The model under review builds one solid part; all positions refer to its coordinate system, in mm. A direction names the side the tool comes from. Give positions to 0.01 mm unless a question says otherwise; leave off trailing zeros. Order: outer loops, then holes, each group sorted by start corner. A loop starts at its lowest first (then second) coordinate and runs counter-clockwise, first axis right, second up.
```python
from build123d import *

# Parameters (mm, degrees)
F0_R     = 11.049
F1_DEPTH = 6.35


with BuildPart() as f1:
    # F0 (on Top) → F1 (new body)
    with BuildSketch(Plane.XY):
        with BuildLine():
            ThreePointArc((-2.36e-08, -13.97), (9.8782817248, -9.8782817415), (13.97, 0))
            ThreePointArc((13.97, 0), (13.8409108955, 1.8947521167), (13.4560292651, 3.754487504))
            ThreePointArc((13.4560292651, 3.754487504), (12.8788953824, 5.4124812914), (12.0983749493, 6.9849998988))
            ThreePointArc((12.0983749493, 6.9849998988), (1.7521013954, 13.8596912195), (-9.9794961892, 9.7760194256))
            ThreePointArc((-9.9794961892, 9.7760194256), (-11.1267940276, 8.4472098748), (-12.0983748995, 6.9849999851))
            ThreePointArc((-12.0983748995, 6.9849999851), (-12.8788953564, -5.4124813532), (-3.4765330758, -13.5305069296))
            ThreePointArc((-3.4765330758, -13.5305069296), (-1.7521013491, -13.8596912254), (-2.36e-08, -13.97))
        make_face()
        Circle(F0_R, mode=Mode.SUBTRACT)
        with BuildLine():
            ThreePointArc((13.4560292651, 3.754487504), (13.8409108955, 1.8947521167), (13.97, 0))
            ThreePointArc((13.97, 0), (9.8782817248, -9.8782817415), (-2.36e-08, -13.97))
            ThreePointArc((-2.36e-08, -13.97), (8.2549999898, -16.1819205776), (14.2980794165, -22.225))
            ThreePointArc((14.2980794165, -22.225), (14.2980794165, -8.255), (26.3964543074, -1.27))
            ThreePointArc((26.3964543074, -1.27), (19.7017499565, 0.1482461704), (14.1572259578, 4.1593236033))
            Line((14.1572259578, 4.1593236033), (13.4560292651, 3.754487504))
        make_face()
        with BuildLine():
            ThreePointArc((12.0983749493, 6.9849998988), (12.8788953824, 5.4124812914), (13.4560292651, 3.754487504))
            Line((13.4560292651, 3.754487504), (14.1572259578, 4.1593236033))
            ThreePointArc((14.1572259578, 4.1593236033), (13.0527933882, 5.5175099241), (12.0983749493, 6.9849998988))
        make_face()
        with BuildLine():
            ThreePointArc((-3.4765330758, -14.3401791282), (-1.7480928878, -14.0628056217), (-2.36e-08, -13.97))
            ThreePointArc((-2.36e-08, -13.97), (-1.7521013491, -13.8596912254), (-3.4765330758, -13.5305069296))
            Line((-3.4765330758, -13.5305069296), (-3.4765330758, -14.3401791282))
        make_face()
        with BuildLine():
            ThreePointArc((-9.9794961892, 9.7760194256), (1.7521013954, 13.8596912195), (12.0983749493, 6.9849998988))
            ThreePointArc((12.0983749493, 6.9849998988), (9.8864543074, 15.2399999416), (12.0983748909, 23.495))
            ThreePointArc((12.0983748909, 23.495), (0, 16.51), (-12.0983748909, 23.495))
            ThreePointArc((-12.0983748909, 23.495), (-9.9792599278, 16.9880928761), (-10.680692882, 10.1808555249))
            Line((-10.680692882, 10.1808555249), (-9.9794961892, 9.7760194256))
        make_face()
        with BuildLine():
            Line((19.5333762679, 7.2632454321), (14.1572259578, 4.1593236033))
            ThreePointArc((14.1572259578, 4.1593236033), (19.7017499565, 0.1482461704), (26.3964543074, -1.27))
            ThreePointArc((26.3964543074, -1.27), (36.2747360405, -5.3617182668), (40.3664543073, -15.24))
            ThreePointArc((40.3664543073, -15.24), (30.0121563674, -28.7339837933), (14.2980794165, -22.225))
            Line((14.2980794165, -22.225), (18.5129530728, -32.0653753202))
            Line((18.5129530728, -32.0653753202), (14.2964770949, -29.5855224255))
            Line((14.2964770949, -29.5855224255), (13.8160917687, -26.1500289008))
            Line((13.8160917687, -26.1500289008), (7.6188843675, -26.0812350595))
            Line((7.6188843675, -26.0812350595), (7.6586053261, -22.5030220397))
            Line((7.6586053261, -22.5030220397), (1.4429174314, -21.1629279691))
            Line((1.4429174314, -21.1629279691), (3.4801004676, -24.6914324922))
            Line((3.4801004676, -24.6914324922), (6.7429192586, -30.342800414))
            Line((6.7429192586, -30.342800414), (12.3789807439, -33.641130461))
            Line((12.3789807439, -33.641130461), (18.9779134399, -37.6940080274))
            Line((18.9779134399, -37.6940080274), (24.2913333671, -32.5875241804))
            Line((24.2913333671, -32.5875241804), (33.0798736321, -35.4493195164))
            Line((33.0798736321, -35.4493195164), (39.4581922442, -29.4734863592))
            Line((39.4581922442, -29.4734863592), (43.9366570858, -23.6116887214))
            Line((43.9366570858, -23.6116887214), (44.0099485225, -16.3618282657))
            Line((44.0099485225, -16.3618282657), (49.9108565981, -16.6858625943))
            Line((49.9108565981, -16.6858625943), (43.1618704508, -11.0453059989))
            Line((43.1618704508, -11.0453059989), (40.7443994954, -2.1940317001))
            Line((40.7443994954, -2.1940317001), (37.0559956245, 4.1944712032))
            Line((37.0559956245, 4.1944712032), (31.3842575072, 5.5065100534))
            Line((31.3842575072, 5.5065100534), (29.1446442552, 12.5378607885))
            Line((29.1446442552, 12.5378607885), (25.7749684952, 7.8452786686))
            Line((25.7749684952, 7.8452786686), (28.8350082813, 4.0347003266))
            Line((28.8350082813, 4.0347003266), (22.6981406857, 4.0953499054))
            Line((22.6981406857, 4.0953499054), (19.5333762679, 7.2632454321))
        make_face()
        with BuildLine():
            Line((-3.4765330758, -14.3401791282), (-3.4765330758, -13.5305069296))
            ThreePointArc((-3.4765330758, -13.5305069296), (-12.8788953564, -5.4124813532), (-12.0983748995, 6.9849999851))
            ThreePointArc((-12.0983748995, 6.9849999851), (-18.1414543148, 0.9419205792), (-26.3964543073, -1.27))
            ThreePointArc((-26.3964543073, -1.27), (-16.5181725742, -5.3617182668), (-12.4264543073, -15.24))
            ThreePointArc((-12.4264543073, -15.24), (-12.9024705141, -18.8557020601), (-14.2980794165, -22.225))
            ThreePointArc((-14.2980794165, -22.225), (-9.7224900287, -17.1363390465), (-3.4765330758, -14.3401791282))
        make_face()
        with BuildLine():
            ThreePointArc((26.3964543074, -1.27), (14.2980794165, -8.255), (14.2980794165, -22.225))
            ThreePointArc((14.2980794165, -22.225), (30.0121563674, -28.7339837933), (40.3664543073, -15.24))
            ThreePointArc((40.3664543073, -15.24), (36.2747360405, -5.3617182668), (26.3964543074, -1.27))
        make_face()
        with Locations((26.3964543073, -15.24)):
            Circle(F0_R, mode=Mode.SUBTRACT)
        with BuildLine():
            Line((-3.4765330758, -20.5480227857), (-3.4765330758, -14.3401791282))
            ThreePointArc((-3.4765330758, -14.3401791282), (-9.7224900287, -17.1363390465), (-14.2980794165, -22.225))
            ThreePointArc((-14.2980794165, -22.225), (-38.4948291982, -22.225), (-26.3964543073, -1.27))
            Line((-26.3964543073, -1.27), (-37.0259061456, 0))
            Line((-37.0259061456, 0), (-32.7700525522, 2.4116488639))
            Line((-32.7700525522, 2.4116488639), (-29.5546352221, 1.1099279977))
            Line((-29.5546352221, 1.1099279977), (-26.3964543073, 6.442470119))
            Line((-26.3964543073, 6.442470119), (-23.3174914114, 4.6189642499))
            Line((-23.3174914114, 4.6189642499), (-19.0490919554, 9.3318608334))
            Line((-19.0490919554, 9.3318608334), (-23.1234580278, 9.3318608334))
            Line((-23.1234580278, 9.3318608334), (-29.6490956098, 9.3318608334))
            Line((-29.6490956098, 9.3318608334), (-35.3235639632, 6.1000534333))
            Line((-35.3235639632, 6.1000534333), (-42.1329252422, 2.4116488639))
            Line((-42.1329252422, 2.4116488639), (-40.3672904702, -4.7431496975))
            Line((-40.3672904702, -4.7431496975), (-47.2399480641, -10.9233511612))
            Line((-47.2399480641, -10.9233511612), (-45.2538840473, -19.4350536913))
            Line((-45.2538840473, -19.4350536913), (-42.4166508019, -26.2444168329))
            Line((-42.4166508019, -26.2444168329), (-36.1747331917, -29.9328193069))
            Line((-36.1747331917, -29.9328193069), (-39.4058091898, -34.8811384415))
            Line((-39.4058091898, -34.8811384415), (-31.146450813, -31.8566232858))
            Line((-31.146450813, -31.8566232858), (-22.2722869366, -34.1886691749))
            Line((-22.2722869366, -34.1886691749), (-14.8954791948, -34.1886691749))
            Line((-14.8954791948, -34.1886691749), (-10.9233511612, -29.9328193069))
            Line((-10.9233511612, -29.9328193069), (-3.7142161756, -31.5089327035))
            Line((-3.7142161756, -31.5089327035), (-6.0932736208, -26.2444168329))
            Line((-6.0932736208, -26.2444168329), (-10.9233511612, -26.9891998532))
            Line((-10.9233511612, -26.9891998532), (-7.8023932874, -21.7048414052))
            Line((-7.8023932874, -21.7048414052), (-3.4765330758, -20.5480227857))
        make_face()
        with BuildLine():
            ThreePointArc((-12.0983748995, 6.9849999851), (-11.1267940276, 8.4472098748), (-9.9794961892, 9.7760194256))
            Line((-9.9794961892, 9.7760194256), (-10.680692882, 10.1808555249))
            ThreePointArc((-10.680692882, 10.1808555249), (-11.3047004812, 8.5452956412), (-12.0983748995, 6.9849999851))
        make_face()
        with BuildLine():
            ThreePointArc((-12.0983748909, 23.495), (0, 16.51), (12.0983748909, 23.495))
            ThreePointArc((12.0983748909, 23.495), (13.4939837933, 26.8642979399), (13.97, 30.48))
            ThreePointArc((13.97, 30.48), (-3.6157020601, 43.9739837933), (-12.0983748909, 23.495))
        make_face()
        with Locations((0, 30.48)):
            Circle(F0_R, mode=Mode.SUBTRACT)
        with BuildLine():
            ThreePointArc((13.97, 30.48), (13.4939837933, 26.8642979399), (12.0983748909, 23.495))
            Line((12.0983748909, 23.495), (18.5129530728, 32.0653753202))
            Line((18.5129530728, 32.0653753202), (18.4735754573, 27.1738735616))
            Line((18.4735754573, 27.1738735616), (15.7385434534, 25.0401009031))
            Line((15.7385434534, 25.0401009031), (18.7775699398, 19.6387649405))
            Line((18.7775699398, 19.6387649405), (15.6588860852, 17.8840577898))
            Line((15.6588860852, 17.8840577898), (17.606174524, 11.8310671357))
            Line((17.606174524, 11.8310671357), (19.6433575602, 15.3595716588))
            Line((19.6433575602, 15.3595716588), (22.9061763512, 21.0109395806))
            Line((22.9061763512, 21.0109395806), (22.9445832193, 27.5410770276))
            Line((22.9445832193, 27.5410770276), (23.1550118023, 35.2823591635))
            Line((23.1550118023, 35.2823591635), (16.0759571031, 37.3306738779))
            Line((16.0759571031, 37.3306738779), (14.160074432, 46.3726706775))
            Line((14.160074432, 46.3726706775), (5.7956918031, 48.9085400505))
            Line((5.7956918031, 48.9085400505), (-1.5200062839, 49.8561055544))
            Line((-1.5200062839, 49.8561055544), (-7.8352153308, 46.2946475726))
            Line((-7.8352153308, 46.2946475726), (-10.5050474083, 51.5670010358))
            Line((-10.5050474083, 51.5670010358), (-12.0154196378, 42.9019292847))
            Line((-12.0154196378, 42.9019292847), (-18.4721125587, 36.382700875))
            Line((-18.4721125587, 36.382700875), (-22.1605164296, 29.9941979717))
            Line((-22.1605164296, 29.9941979717), (-20.460906346, 24.4263092535))
            Line((-20.460906346, 24.4263092535), (-25.4304280796, 18.971071915))
            Line((-25.4304280796, 18.971071915), (-19.6816948744, 18.3991381643))
            Line((-19.6816948744, 18.3991381643), (-17.9116571201, 22.9544995267))
            Line((-17.9116571201, 22.9544995267), (-14.8957473983, 17.6094914998))
            Line((-14.8957473983, 17.6094914998), (-16.0568431921, 13.2847773536))
            Line((-16.0568431921, 13.2847773536), (-10.680692882, 10.1808555249))
            ThreePointArc((-10.680692882, 10.1808555249), (-9.9792599278, 16.9880928761), (-12.0983748909, 23.495))
            ThreePointArc((-12.0983748909, 23.495), (-3.6157020601, 43.9739837933), (13.97, 30.48))
        make_face()
        with BuildLine():
            ThreePointArc((-26.3964543073, -1.27), (-38.4948291982, -22.225), (-14.2980794165, -22.225))
            ThreePointArc((-14.2980794165, -22.225), (-12.9024705141, -18.8557020601), (-12.4264543073, -15.24))
            ThreePointArc((-12.4264543073, -15.24), (-16.5181725742, -5.3617182668), (-26.3964543073, -1.27))
        make_face()
        with Locations((-26.3964543073, -15.24)):
            Circle(F0_R, mode=Mode.SUBTRACT)
    extrude(amount=F1_DEPTH)


solid = f1.part
```
Item 1: Draft analysis for pull direction Y (two halves, no side actions). For faces 5 (the flat face through (-11.25, 47.3, 3.13)), 6 (the flat face through (36.224, -32.503, 3.131)), 7 (the flat face through (16.376, -27.076, 3.131)), state which applies: released by +Y, released by -Y, zero draft, split by the parting line, or undercut.
Values found:
face 5: released by +Y
face 6: released by -Y
face 7: undercut
Item 2: Take a section at C-C (z = 1.75). Give the number of separate pieces and of enclosed holes in the cut face, and give its area (3 significant figures).
Values found:
separate pieces: 1
enclosed holes: 4
area: 2,840 mm2
Item 3: Take a section at B-B (y = 40). Give the boundary of the cut face in (x, z).
Values found:
outline: (-14.89, 0) - (-5.61, 0) - (-5.61, 6.35) - (-14.89, 6.35) - close; (5.61, 0) - (15.51, 0) - (15.51, 6.35) - (5.61, 6.35) - close
Item 4: Clearance check with flat-ended pins moving along their axes: pin 1 Ø20 at (x, y) = (26.4, -15.24) entering from -Z; pin 2 Ø12 at (x, y) = (-13.5, 11.5) entering from +Z; pin 3 Ø1.9 at (y, z) = (-18, 3.5) entering from +X; pin 4 Ø2 at (y, z) = (8.5, 5) entering from -X. State where each tip first meets the part, or that it passes through.
Values found:
pin 1: passes through
pin 2: stops at z = 6.35
pin 3: stops at x = 44
pin 4: stops at x = -32.87
Item 5: Take a section at A-A (y = -6.5). Give the boundary of the cut face in (x, z), and give its area (3 significant figures).
Values found:
outline: (-42.32, 0) - (-33.16, 0) - (-33.16, 6.35) - (-42.32, 6.35) - close; (-19.64, 0) - (-8.93, 0) - (-8.93, 6.35) - (-19.64, 6.35) - close; (8.93, 0) - (19.64, 0) - (19.64, 6.35) - (8.93, 6.35) - close; (33.16, 0) - (41.92, 0) - (41.92, 6.35) - (33.16, 6.35) - close
area: 250 mm2
Item 6: For line 1 (X direction, y = 29, z = 6.25); line 2 (X direction, y = -27.5, z = 1.75); line 3 (Y direction, x = 0, z = 4.75), list the stretches that pass through material, from the lowest coordinate up.
Values found:
line 1: x = -21.86 to -10.95, 10.95 to 16.22, 18.49 to 22.98
line 2: x = -40.29 to -5.53, 5.1 to 14, 16.56 to 40.97
line 3: y = -13.97 to -11.05, 11.05 to 19.43, 41.53 to 49.66
Item 7: For faces 1 (the flat face through (-19, -34.189, 3)), 2 (the flat face through (-4.63, 48.1, 3.13)), 3 (the flat face through (-31.18, 1.77, 3.13)), 4 (the flat face through (-41.26, -1.12, 3.13)), list the 3-axis set-ups (+Z, -Z, +X, -X, +Y, -Y) from which the entire face can be reached by the end or side of a thin tool; tool diameter is ignored.
Values found:
face 1: +Z, -Z, -Y
face 2: +Z, -Z, +Y
face 3: +Z, -Z
face 4: +Z, -Z, -X
